Can you work these out from the model? Positions are in its coordinate system, mm. A direction names the side the tool comes from. Round coordinates to 2 decimals unless told otherwise and drop trailing zeros. Loops run counter-clockwise (first coordinate to the right, second up) from the corner with the lowest first, then second, coordinate; pieces in that order, holes last. Notation, with made-up numbers: (-35.5, 0) -> (-16.5, 0) arc R22 cw to (-16.5, 37) -> close; hole circle Ø10 at (24, -9). An arc over 180 degrees is marked (long way). Write item = value, one per line.
Solid Edge part; units mm, degrees
sketch "Sketch1" plane through (0, 0, 0) normal (0, 0, 1) x (1, 0, 0)
  line L0 (-1.5, 38) -> (-37.5, 38)
  line L1 (-37.5, 38) -> (-37.5, 29)
  line L2 (-37.5, 29) -> (-33.5, 29)
  line L3 (-33.5, 29) -> (-33.5, 34)
  line L4 (-33.5, 34) -> (-30.9, 34)
  line L5 (-30.9, 34) -> (-30.9, 29)
  line L6 (-30.9, 29) -> (-26.9, 29)
  line L7 (-26.9, 29) -> (-26.9, 34)
  line L8 (-26.9, 34) -> (-5.5, 34)
  line L9 (-5.5, 34) -> (-5.5, 0)
  line L10 (-5.5, 0) -> (0, 0)
  line L11 (0, 0) -> (0, 10)
  line L12 (0, 10) -> (-1.5, 24.2715)
  line L13 (-1.5, 24.2715) -> (-1.5, 38)
  dimension "D1" = 37.5
  dimension "D2" = 5.5
  dimension "D3" = 33.5
  dimension "D4" = 33.5
  dimension "D5" = 30.9
  dimension "D6" = 5.5
extrude "Protrusion1" add sketch "Sketch1" along normal mid plane 12
hole "Agujero_1" at (-37.5, 31, 0) direction (1, 0, 0) diameter 2 depth 19.6879
hole "Agujero_3" at (-5.5, 3.5, 0) direction (1, 0, 0) diameter 2 end up to next
chamfer "Chaflán_1" distance 1 angle 45 2 edges at (-37.5, 31, -1) (0, 4.5, 0)
fillet "Redondeo_4" radius 10 1 edges at (-5.5, 34, 0)
fillet "Redondeo_5" radius 2 1 edges at (-26.9, 34, 0)
fillet "Redondeo_2" radius 4 1 edges at (-37.5, 38, 0)
fillet "Redondeo_3" radius 2 2 edges at (-2.75, 0, 6) (-2.75, 0, -6)
fillet "Redondeo_6" radius 14 1 edges at (-1.5, 38, 0)
hole "Agujero_4" at (0, 13.5, 0) direction (-1, 0, 0) diameter 6.1 end up to next
properties material "ABS, medio impacto"
1. Suppose I cut it at D-D, the plane z = 0. Count the separate pieces of the cut face and the enclosed holes in it, and give its area (3 significant figures).
Entries:
separate_pieces = 5
enclosed_holes = 0
area = 262 mm²
2. We'd pull the mould along Z, two halves only. Please class faces 4 (the cylindrical face through (-26.3, 33.43, 0.08)), 5 (the cylindrical face through (-2.71, 0.57, -5.4)), 6 (the cylindrical face through (-35, 30, 0)): released by +Z, released by -Z, zero draft, split by the parting line, or undercut.
Entries:
face_4 = zero draft
face_5 = released by -Z
face_6 = undercut
3. For faces 1 (the flat face through (-32, 34, 0)), 2 (the flat face through (-36, 29, 0)), 3 (the cylindrical face through (-2.735, 10.794, -1.407)), which set-ups out of +Z, -Z, +X, -X, +Y, -Y let a thin tool reach every point of the face, with its end or its side?
Entries:
face_1 = +Z, -Z, -Y
face_2 = +Z, -Z, -X, -Y
face_3 = +X, -X
4. I'm going to push flat-ended pins straight in: pin 1 (1.2 mm diameter, centred on y = 3.5, z = 0, fed in from -X); pin 2 (6 mm diameter, centred on y = 10.5, z = 2, fed in from -X); pin 3 (1.2 mm diameter, centred on x = -29, z = 0.5, fed in from -Y); pin 4 (1.2 mm diameter, centred on y = 31, z = 0, fed in from +X). Where does each tip first touch, or does it pass through?
Entries:
pin_1 = through
pin_2 = -5.5
pin_3 = 29
pin_4 = -3.05
5. Suppose I cut it at A-A, the plane y = 3.5. List the corners of the cut face in (x, z) for me, and give its area (3 significant figures).
Entries:
outline = (-5.5, -6) -> (0, -6) -> (0, -2) -> (-1, -1) -> (-5.5, -1) -> close; (-5.5, 1) -> (-1, 1) -> (0, 2) -> (0, 6) -> (-5.5, 6) -> close
area = 54.0 mm²
6. I need wall thicknesses on line 1 (Z direction, x = -29.7, y = 31); line 2 (X direction, y = 30, z = -4); line 3 (Y direction, x = -2.6, z = 0). Which ranges of each line are inside material? Lowest first, please. Write a range as [from, to].
Entries:
line_1 = [-6, -1], [1, 6]
line_2 = [-37.5, -33.5], [-30.9, -26.9], [-7.5, -2.85]
line_3 = [0, 2.5], [4.5, 10.45], [16.55, 29.44]
7. Suppose I cut it at C-C, the plane x = -21.5. List the corners of the cut face in (y, z) for me, and give its area (3 significant figures).
Entries:
outline = (34, -6) -> (38, -6) -> (38, 6) -> (34, 6) -> close
area = 48.0 mm²
8. Suppose I cut it at B-B, the plane y = 31. List the corners of the cut face in (x, z) for me.
Entries:
outline = (-37.5, -6) -> (-33.5, -6) -> (-33.5, -1) -> (-36.5, -1) -> (-37.5, -2) -> close; (-37.5, 2) -> (-36.5, 1) -> (-33.5, 1) -> (-33.5, 6) -> (-37.5, 6) -> close; (-30.9, -6) -> (-26.9, -6) -> (-26.9, -1) -> (-30.9, -1) -> close; (-30.9, 1) -> (-26.9, 1) -> (-26.9, 6) -> (-30.9, 6) -> close; (-8.36, -6) -> (-3.38, -6) -> (-3.38, 6) -> (-8.36, 6) -> close
